from build123d import *

# Parameters (mm, degrees)
SKETCH1_W           = 144.5
SKETCH1_H           = 100
SKETCH1_R           = 1.55
BOSS_EXTRUDE1_DEPTH = 2.8
CUT_EXTRUDE1_REACH  = 4.8
SKETCH2_R           = 1.55
CUT_EXTRUDE2_REACH  = 4.8
SKETCH3_R           = 1.55


with BuildPart() as part:
    # Sketch1 → Boss-Extrude1 (new body)
    with BuildSketch(Plane(origin=(0, 0, 0), x_dir=(1, 0, 0), z_dir=(0, 1, 0))):
        Rectangle(SKETCH1_W, SKETCH1_H)
        with Locations((-32.25, 40)):
            Circle(SKETCH1_R, mode=Mode.SUBTRACT)
        with Locations((59.25, 20)):
            Circle(SKETCH1_R, mode=Mode.SUBTRACT)
        with Locations((42.25, -40)):
            Circle(SKETCH1_R, mode=Mode.SUBTRACT)
    extrude(amount=BOSS_EXTRUDE1_DEPTH)

    # Sketch2 → Cut-Extrude1 (cut, up to next)
    with BuildSketch(Plane(origin=(0, 2.8, 0), x_dir=(1, 0, 0), z_dir=(0, 1, 0)), mode=Mode.PRIVATE) as cut_extrude1_sk1:
        with Locations((-36.75, -21.73)):
            Circle(SKETCH2_R)
    cut_extrude1_tool1 = extrude(cut_extrude1_sk1.sketch, amount=-CUT_EXTRUDE1_REACH, mode=Mode.PRIVATE) & part.part
    add(cut_extrude1_tool1.solids().sort_by_distance((-36.75, 2.8, 21.73))[0], mode=Mode.SUBTRACT)

    # Sketch3 → Cut-Extrude2 (cut, up to next)
    with BuildSketch(Plane(origin=(0, 2.8, 0), x_dir=(1, 0, 0), z_dir=(0, 1, 0)), mode=Mode.PRIVATE) as cut_extrude2_sk1:
        with Locations((37.999537704, 15.380946094)):
            Circle(SKETCH3_R)
    cut_extrude2_tool1 = extrude(cut_extrude2_sk1.sketch, amount=-CUT_EXTRUDE2_REACH, mode=Mode.PRIVATE) & part.part
    add(cut_extrude2_tool1.solids().sort_by_distance((37.999538, 2.8, -15.380946))[0], mode=Mode.SUBTRACT)
    # Sketch3 → Cut-Extrude2 (cut, up to next)
    with BuildSketch(Plane(origin=(0, 2.8, 0), x_dir=(1, 0, 0), z_dir=(0, 1, 0)), mode=Mode.PRIVATE) as cut_extrude2_sk2:
        with Locations((45.25, 12)):
            Circle(SKETCH3_R)
    cut_extrude2_tool2 = extrude(cut_extrude2_sk2.sketch, amount=-CUT_EXTRUDE2_REACH, mode=Mode.PRIVATE) & part.part
    add(cut_extrude2_tool2.solids().sort_by_distance((45.25, 2.8, -12))[0], mode=Mode.SUBTRACT)


solid = part.part
CAD build for the part. Positions are in the model's coordinates, mm. Coordinates: 2 decimals unless noted, no trailing zeros. Write each loop counter-clockwise with the first axis right and the second up, starting at its lowest first coordinate (ties: lowest second). Pieces come first, ordered by that corner, then holes. Notation, with made-up numbers: M -12.75,37 L 14.25,37 A22 ccw 14.25,60 Z; hole C -26,-26 d4. An arc over 180 degrees is marked long. Answer as a JSON object with one key per item and string values. Group by question number.
1) Saw through at A-A (x = 45.25). Write the cut outline in (y, z), plus the area to 3 significant figures.
2) Wall check: line 1 (Z direction, x = 42.25, y = 1.1); line 2 (X direction, y = 1.3, z = -12); line 3 (X direction, y = 1, z = 40). Give the ranges that are in metal, low to high. Write a range as from..to.
3) Saw through at B-B (z = -40). Write the cut outline in (x, y).
4) Pin check, flat tip, straight feed: pin 1 Ø1.9 at (x, z) = (42.25, 40) entering from +Y. Stop position of the tip, or through.
5) Mould opens along Z. For faces 1 (the face through (36.86, 1.42, -16.43)), 2 (the face through (-1, 2.8, -1)), 3 (the face through (-1, 1, -50)) say: +Z half, -Z half, draft (parallel to the pull), parting line (faces both ways), or undercut.
Values follow:
{
 "1": {"outline": "M 0,-50 L 2.8,-50 L 2.8,-13.55 L 0,-13.55 Z; M 0,-10.45 L 2.8,-10.45 L 2.8,50 L 0,50 Z", "area": "271 mm2"},
 "2": {"line 1": "z = -50..38.45, 41.55..50", "line 2": "x = -72.25..43.7, 46.8..72.25", "line 3": "x = -72.25..40.7, 43.8..72.25"},
 "3": {"outline": "M -72.25,0 L -33.8,0 L -33.8,2.8 L -72.25,2.8 Z; M -30.7,0 L 72.25,0 L 72.25,2.8 L -30.7,2.8 Z"},
 "4": {"pin 1": "passes through"},
 "5": {"face 1": "undercut", "face 2": "draft", "face 3": "-Z half"}
}
